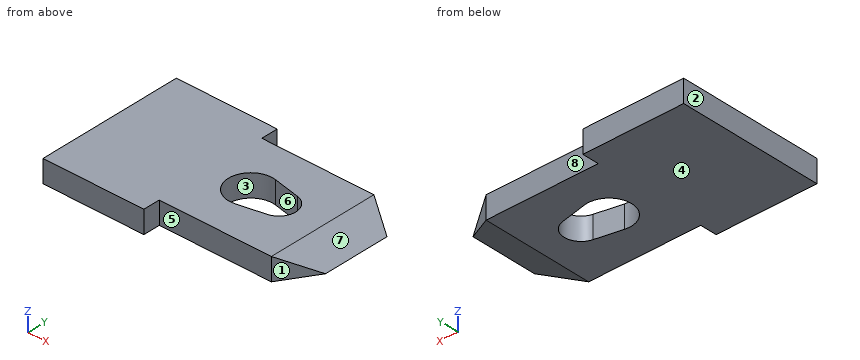
from build123d import *

# Parameters (mm, degrees)
DODANIE_WYCI_GNI_CIE1_DEPTH = 1
WYTNIJ_WYCI_GNI_CIE1_REACH  = 3
WYTNIJ_WYCI_GNI_CIE2_REACH  = 7.75


with BuildPart() as part:
    # Szkic1 → Dodanie-wyciągnięcie1 (new body)
    with BuildSketch(Plane.XY):
        Polygon((0, -3.25), (0, 3.25), (4.5, 3.25), (4.5, 2.5), (9.5, 2.5), (11, 1.5), (11, -1.5), (9.5, -2.5), (4.5, -2.5), (4.5, -3.25), align=None)
    extrude(amount=DODANIE_WYCI_GNI_CIE1_DEPTH)

    # Szkic2 → Wytnij-wyciągnięcie1 (cut, up to next)
    with BuildSketch(Plane.XY.offset(1), mode=Mode.PRIVATE) as wytnij_wyci_gni_cie1_sk1:
        with BuildLine():
            Line((6.5, 0.979795897), (7.7, 0.734846923))
            ThreePointArc((7.7, 0.734846923), (8.3, 0), (7.7, -0.734846923))
            Line((7.7, -0.734846923), (6.5, -0.979795897))
            ThreePointArc((6.5, -0.979795897), (5.3, 0), (6.5, 0.979795897))
        make_face()
    wytnij_wyci_gni_cie1_tool1 = extrude(wytnij_wyci_gni_cie1_sk1.sketch, amount=-WYTNIJ_WYCI_GNI_CIE1_REACH, mode=Mode.PRIVATE) & part.part
    add(wytnij_wyci_gni_cie1_tool1.solids().sort_by_distance((6.737463, 0, 1))[0], mode=Mode.SUBTRACT)

    # Szkic3 → Wytnij-wyciągnięcie2 (cut, up to next)
    with BuildSketch(Plane(origin=(0, 2.5, 0), x_dir=(1, 0, 0), z_dir=(0, 1, 0)), mode=Mode.PRIVATE) as wytnij_wyci_gni_cie2_sk1:
        Polygon((11, -1), (11, -0.5), (9.5, -1), align=None)
    wytnij_wyci_gni_cie2_tool1 = extrude(wytnij_wyci_gni_cie2_sk1.sketch, amount=-WYTNIJ_WYCI_GNI_CIE2_REACH, mode=Mode.PRIVATE) & part.part
    add(wytnij_wyci_gni_cie2_tool1.solids().sort_by_distance((10.5, 2.5, 0.833333))[0], mode=Mode.SUBTRACT)
    # Szkic3 → Wytnij-wyciągnięcie2 (cut, up to next)
    with BuildSketch(Plane(origin=(0, 2.5, 0), x_dir=(1, 0, 0), z_dir=(0, 1, 0)), mode=Mode.PRIVATE) as wytnij_wyci_gni_cie2_sk2:
        Polygon((9.5, 0), (11, -0.5), (11, 0), align=None)
    wytnij_wyci_gni_cie2_tool2 = extrude(wytnij_wyci_gni_cie2_sk2.sketch, amount=-WYTNIJ_WYCI_GNI_CIE2_REACH, mode=Mode.PRIVATE) & part.part
    add(wytnij_wyci_gni_cie2_tool2.solids().sort_by_distance((10.5, 2.5, 0.166667))[0], mode=Mode.SUBTRACT)


solid = part.part
For this review, take the finished solid that the model builds, in its own axes (mm). Face numbers are marked on the shaded views. A direction names the side the tool comes from. Round coordinates to 2 decimals unless told otherwise and drop trailing zeros. Order: outer loops, then holes, each group sorted by start corner. A loop starts at its lowest first (then second) coordinate and runs counter-clockwise, first axis right, second up. Notation, with made-up numbers: (67.5, 81.5) -> (108.5, 81.5) arc R7 ccw to (108.5, 90.5) -> close; hole circle Ø1 at (-19.5, -24). An arc over 180 degrees is marked (long way). Write item = value, one per line. Start each with the question number.
1) The part is to be moulded in two halves that separate along Y. For the marked faces 1, 2 and 3, say which applies: +Y half, -Y half, draft (parallel to the pull), parting line (faces both ways), or undercut.
2) Tool access review of the marked faces 4, 5, 6, 7 and 8: name each direction out of +Z, -Z, +X, -X, +Y, -Y from which nothing blocks a thin tool from reaching the whole face with its end or side.
3) Take a section at D-D on y = 2. State the section outline as (x, z) points, plus the area to 3 significant figures.
4) Take a section at C-C on z = 0.7. State the section outline as (x, y) points.
5) To check wall thickness, follow line 1 (Y direction, x = 6.3, z = 0.8); line 2 (X direction, y = 2.75, z = 0.45); line 3 (Y direction, x = 8, z = 0.4). State the ranges of each line that lie inside material, in increasing order. Write a range as from..to.
6) Take a section at B-B on x = 6.3. State the section outline as (y, z) points, plus the area to 3 significant figures.
7) Take a section at A-A on y = 0. State the section outline as (x, z) points.
Verdict:
q1.face_1 = -Y half
q1.face_2 = draft
q1.face_3 = undercut
q2.face_4 = -Z, +X, -X, +Y, -Y
q2.face_5 = +Z, -Z, +X, -Y
q2.face_6 = +Z, -Z
q2.face_7 = +Z, +X, +Y, -Y
q2.face_8 = +Z, -Z, +X, +Y
q3.outline = (0, 0) -> (9.5, 0) -> (10.25, 0.25) -> (10.25, 0.75) -> (9.5, 1) -> (0, 1) -> close
q3.area = 10.1 mm2
q4.outline = (0, -3.25) -> (4.5, -3.25) -> (4.5, -2.5) -> (9.5, -2.5) -> (10.4, -1.9) -> (10.4, 1.9) -> (9.5, 2.5) -> (4.5, 2.5) -> (4.5, 3.25) -> (0, 3.25) -> close; hole (6.5, -0.98) -> (7.7, -0.73) arc R0.75 ccw to (7.7, 0.73) -> (6.5, 0.98) arc R1 ccw (long way) to start
q5.line_1 = -2.5..-1, 1..2.5
q5.line_2 = 0..4.5
q5.line_3 = -2.5..-0.6, 0.6..2.5
q6.outline = (-2.5, 0) -> (-1, 0) -> (-1, 1) -> (-2.5, 1) -> close; (1, 0) -> (2.5, 0) -> (2.5, 1) -> (1, 1) -> close
q6.area = 3.00 mm2
q7.outline = (0, 0) -> (5.3, 0) -> (5.3, 1) -> (0, 1) -> close; (8.3, 0) -> (9.5, 0) -> (11, 0.5) -> (9.5, 1) -> (8.3, 1) -> close
